from build123d import *

# Parameters (mm, degrees)
SKETCH1_W           = 9.525
SKETCH1_H           = 25.4
BOSS_EXTRUDE1_DEPTH = 4.7625
CUT_EXTRUDE1_REACH  = 18.574
SKETCH2_W           = 3.175
SKETCH2_H           = 21.59
CUT_EXTRUDE2_REACH  = 18.574
SKETCH3_R           = 2.159
CUT_EXTRUDE3_REACH  = 28.278
SKETCH4_W           = 5.461
SKETCH4_H           = 1.016
SKETCH5_W           = 1.016
SKETCH5_H           = 19.558
CUT_EXTRUDE4_DEPTH  = 17.573986583


with BuildPart() as part:
    # Sketch1 → Boss-Extrude1 (new, symmetric)
    with BuildSketch(Plane.XY):
        Rectangle(SKETCH1_W, SKETCH1_H)
    extrude(amount=BOSS_EXTRUDE1_DEPTH, both=True)

    # Sketch2 → Cut-Extrude1 (cut, up to next)
    with BuildSketch(Plane(origin=(4.7625, 0, 0), x_dir=(0, 0, -1), z_dir=(1, 0, 0)), mode=Mode.PRIVATE) as cut_extrude1_sk1:
        with Locations((3.175, -1.905)):
            Rectangle(SKETCH2_W, SKETCH2_H)
    cut_extrude1_tool1 = extrude(cut_extrude1_sk1.sketch, amount=-CUT_EXTRUDE1_REACH, mode=Mode.PRIVATE) & part.part
    add(cut_extrude1_tool1.solids().sort_by_distance((4.7625, -1.905, -3.175))[0], mode=Mode.SUBTRACT)

    # Sketch3 → Cut-Extrude2 (cut, up to next)
    with BuildSketch(Plane.XY.offset(4.7625), mode=Mode.PRIVATE) as cut_extrude2_sk1:
        with Locations((1.5875, -1.27)):
            Circle(SKETCH3_R)
    cut_extrude2_tool1 = extrude(cut_extrude2_sk1.sketch, amount=-CUT_EXTRUDE2_REACH, mode=Mode.PRIVATE) & part.part
    add(cut_extrude2_tool1.solids().sort_by_distance((1.5875, -1.27, 4.7625))[0], mode=Mode.SUBTRACT)

    # Sketch4 → Cut-Extrude3 (cut, up to next)
    with BuildSketch(Plane(origin=(0, 12.7, 0), x_dir=(1, 0, 0), z_dir=(0, 1, 0)), mode=Mode.PRIVATE) as cut_extrude3_sk1:
        with Locations((0, 4.2545)):
            Rectangle(SKETCH4_W, SKETCH4_H)
    cut_extrude3_tool1 = extrude(cut_extrude3_sk1.sketch, amount=-CUT_EXTRUDE3_REACH, mode=Mode.PRIVATE) & part.part
    add(cut_extrude3_tool1.solids().sort_by_distance((0, 12.7, -4.2545))[0], mode=Mode.SUBTRACT)

    # Sketch5 → Cut-Extrude4 (cut, through all)
    with BuildSketch(Plane(origin=(4.7625, 0, 0), x_dir=(0, 0, -1), z_dir=(1, 0, 0))):
        with Locations((1.0795, -0.889)):
            Rectangle(SKETCH5_W, SKETCH5_H)
    extrude(amount=-CUT_EXTRUDE4_DEPTH, mode=Mode.SUBTRACT)


solid = part.part
Work out the finished part from the listing and answer in its coordinate system (mm). A direction names the side the tool comes from. Coordinates: 2 decimals unless noted, no trailing zeros. Loops run counter-clockwise (first coordinate to the right, second up) from the corner with the lowest first, then second, coordinate; pieces in that order, holes last. Notation, with made-up numbers: (-38.5, -11.5) -> (-7.5, -11.5) arc R16 cw to (-7.5, 15.5) -> close; hole circle Ø11 at (43.5, 51). An arc over 180 degrees is marked (long way). Answer as CSV lines item,"result".
1) For a pull along Y with two mould halves and no side action, classify faces 1 (the face through (0, 8.89, -3)), 2 (the face through (0, -12.7, 2)), 3 (the face through (-1, 0, 4.762)) as released by +Y, released by -Y, zero draft, split by the parting line, or undercut.
A:
face 1,"undercut"
face 2,"released by -Y"
face 3,"zero draft"
2) The part is cut by section B-B (x = 3). Give the vertices of the cut face in (y, z), and give its area (3 significant figures).
A:
outline,"(-12.7, -1.59) -> (-10.67, -1.59) -> (-10.67, -0.57) -> (-2.9, -0.57) -> (-2.9, 4.76) -> (-12.7, 4.76) -> close; (0.36, -0.57) -> (8.89, -0.57) -> (8.89, -4.76) -> (12.7, -4.76) -> (12.7, 4.76) -> (0.36, 4.76) -> close"
area,"136 mm²"
3) The part is cut by section A-A (y = -1.27). Give the vertices of the cut face in (x, z), and give its area (3 significant figures).
A:
outline,"(-4.76, -0.57) -> (-0.57, -0.57) -> (-0.57, 4.76) -> (-4.76, 4.76) -> close; (3.75, -0.57) -> (4.76, -0.57) -> (4.76, 4.76) -> (3.75, 4.76) -> close"
area,"27.8 mm²"
4) Straight lines are drawn through the part: probe 1 along Y at (x, z) = (1, -0.75); probe 2 along Z at (x, y) = (-1.25, 8.25); probe 3 along Y at (x, z) = (-0.75, -3.25). For each, find the intervals that lie inside material, in ascending order.
A:
probe 1,"y = -12.7 to -10.67, 8.89 to 12.7"
probe 2,"z = -0.57 to 4.76"
probe 3,"y = 8.89 to 12.7"
5) Flat-ended cylindrical pins translate along their axes: pin 1 (1.3 mm diameter, centred on x = 2, z = -2.5, fed in from -Y); pin 2 (0.6 mm diameter, centred on x = -0.5, y = -11.5, fed in from -Z); pin 3 (3 mm diameter, centred on x = -1, y = -3.5, fed in from -Z). Find the tip coordinate at first contact, or state that the pin passes through.
A:
pin 1,"stops at y = 8.89"
pin 2,"stops at z = -1.59"
pin 3,"stops at z = -0.57"
6) The part is cut by section C-C (z = -1). Give the vertices of the cut face in (x, y), and give its area (3 significant figures).
A:
outline,"(-4.76, -12.7) -> (4.76, -12.7) -> (4.76, -10.67) -> (-4.76, -10.67) -> close; (-4.76, 8.89) -> (4.76, 8.89) -> (4.76, 12.7) -> (-4.76, 12.7) -> close"
area,"55.6 mm²"
7) For faces 4 (the face through (-0.13, -2.58, 2.13)), 5 (the face through (-2.73, 11, -4)), 6 (the face through (0, -12, -1.588)), 7 (the face through (0, -10.668, -1)), determine the directions among +Z, -Z, +X, -X, +Y, -Y from which every point of the face is accessible in a straight line to the end or side of a thin tool.
A:
face 4,"+Z, -Z"
face 5,"-Z, +Y, -Y"
face 6,"-Z, +X, -X, -Y"
face 7,"-Z, +X, -X"
8) The part is cut by section D-D (y = 6.25). Give the vertices of the cut face in (x, z), and give its area (3 significant figures).
A:
outline,"(-4.76, -0.57) -> (4.76, -0.57) -> (4.76, 4.76) -> (-4.76, 4.76) -> close"
area,"50.8 mm²"
